For this review, use the dimensioned drawing (mm, ordinates from the lowest corner) and the shaded views. Round coordinates to 2 decimals unless told otherwise and drop trailing zeros. Write each loop counter-clockwise with the first axis right and the second up, starting at its lowest first coordinate (ties: lowest second). Pieces come first, ordered by that corner, then holes. Notation, with made-up numbers: (27, 3.25) - (47, 3.25) arc R6 cw to (47, 14.25) - close; hole circle Ø1 at (-5, 35.5). An arc over 180 degrees is marked (long way). Write each question's results on one line, items separated by ' | '.
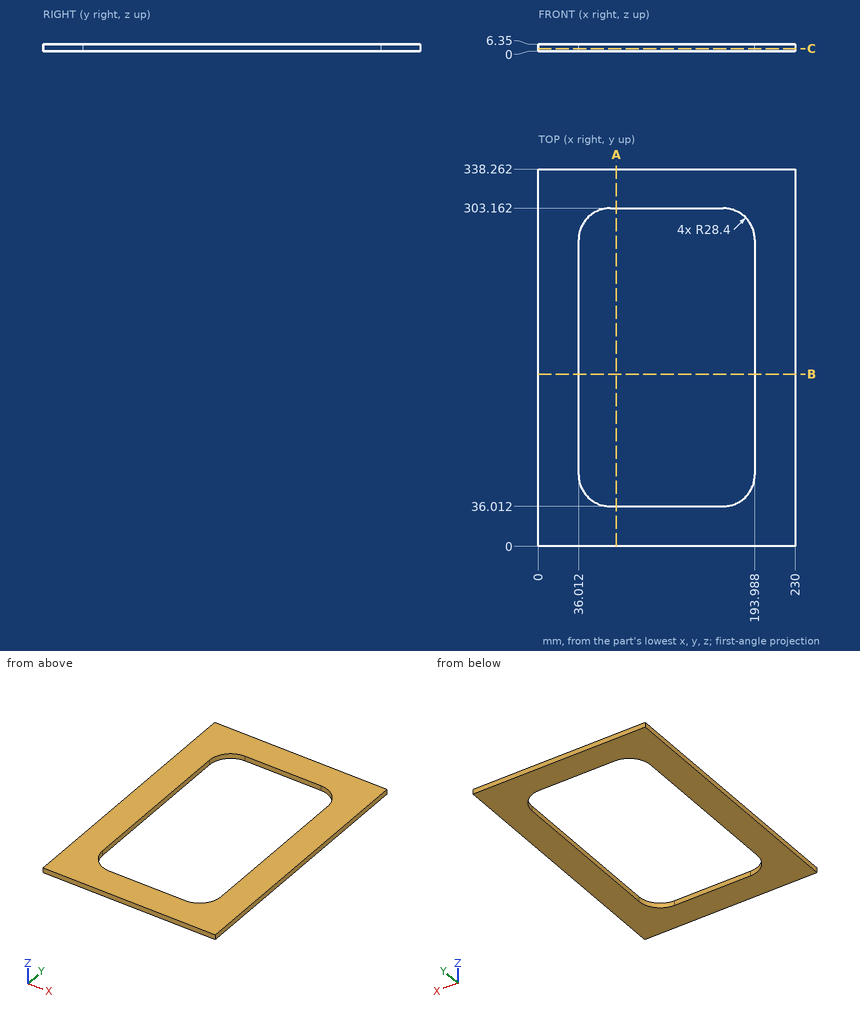
Q1. We need section B-B (y = 154.5). State the section outline as (x, z) points.
Evaluation:
outline: (0, 0) - (36.01, 0) - (36.01, 6.35) - (0, 6.35) - close; (193.99, 0) - (230, 0) - (230, 6.35) - (193.99, 6.35) - close
Q2. We need section A-A (x = 70). State the section outline as (y, z) points, plus the area to 3 significant figures.
Evaluation:
outline: (0, 0) - (36.01, 0) - (36.01, 6.35) - (0, 6.35) - close; (303.16, 0) - (338.26, 0) - (338.26, 6.35) - (303.16, 6.35) - close | area: 452 mm^2
Q3. We need section C-C (z = 2.25). State the section outline as (x, y) points.
Evaluation:
outline: (0, 0) - (230, 0) - (230, 338.26) - (0, 338.26) - close; hole (36.01, 64.41) arc R28.4 ccw to (64.41, 36.01) - (165.59, 36.01) arc R28.4 ccw to (193.99, 64.41) - (193.99, 274.76) arc R28.4 ccw to (165.59, 303.16) - (64.41, 303.16) arc R28.4 ccw to (36.01, 274.76) - close
Q4. For probe 1 along X at (y, z) = (206, 4.25); probe 2 along Y at (x, z) = (147, 2.5); probe 3 along Y at (x, z) = (39.5, 2.75), list the stretches that pass through material, from the lowest coordinate up.
Evaluation:
probe 1: x = 0 to 36.01, 193.99 to 230 | probe 2: y = 0 to 36.01, 303.16 to 338.26 | probe 3: y = 0 to 50.78, 288.4 to 338.26
